Can you work these out from the model? Positions are in its coordinate system, mm. A direction names the side the tool comes from. Give positions to 0.01 mm unless a question says otherwise; leave off trailing zeros. Write each loop counter-clockwise with the first axis right and the second up, starting at its lowest first coordinate (ties: lowest second). Pieces come first, ordered by that corner, then holes. Notation, with made-up numbers: (70, 0.25) -> (92, 0.25) arc R29 cw to (92, 22.25) -> close; hole circle Ø4 at (-5, -26). An arc over 180 degrees is marked (long way). Answer as CSV lines item,"result". Start each with the question number.
1. I'm going to push flat-ended pins straight in: P1, Ø12, axis at x = 3.5, y = -3, coming from the -Z side; P2, Ø12, axis at x = -11.5, z = -21.5, coming from the -Y side; P3, Ø2.5, axis at x = 5.5, z = 1, coming from the +Y side. Where does each tip first touch, or does it pass through?
2. If we section it at D-D on y = -17.5: Write out the boundary of the cut face in (x, z) (3 decimals), plus the area to 3 significant figures.
3. If we mould it in two halves opening along Z, with no side actions, what happens to faces 6 (the face through (-1.032, 16.25, -11.226)), 7 (the face through (21.31, 0.73, -4.7)), 8 (the face through (18.573, -5.104, 1.565))? For each: pulls with the +Z half, pulls with the -Z half, needs draft (parallel to the pull), parting line crosses it, or undercut.
4. I need wall thicknesses on line 1 (Z direction, x = 0, y = 7.35) (3 decimals); line 2 (Z direction, x = 0, y = 18) (1 decimal); line 3 (Z direction, x = -15, y = -16) (3 decimals). Which ranges of each line are inside material? Lowest first, please. Write a range as [from, to].
5. On a 3-axis mill with a long thin cutter (end or side, diameter ignored), from which of +Z, -Z, +X, -X, +Y, -Y can I reach the whole of each face in a straight line? I mean faces 1 (the face through (0, -14, 0)), 2 (the face through (1, 8.458, -18.1)), 3 (the face through (0.49, 6.99, -13.68)), 4 (the face through (-19.05, 1, -1)), 5 (the face through (-0.33, 17.78, -31.44)). Say none if no direction works.
6. If we section it at A-A on x = 0: Count the separate pieces of the cut face and the enclosed holes in it, plus the area to 3 significant figures.
7. If we section it at B-B on y = 1: Write out the boundary of the cut face in (x, z) (3 decimals).
```python
from build123d import *
from build123d.topology import SkipClean

# Parameters (mm, degrees)
SKETCH1_R                                           = 23.8252
BOSS_EXTRUDE1_DEPTH                                 = 3.175
SKETCH8_W                                           = 38.1
SKETCH8_H                                           = 11.1125
CUT_EXTRUDE1_DEPTH                                  = 34.843181515
FILLET1_R                                           = 1.5875
BOSS_EXTRUDE2_START                                 = 31.75
BOSS_EXTRUDE2_DEPTH                                 = 31.75
CHAMFER1_START                                      = -23.8252001
CHAMFER1_DEPTH                                      = 6.3627001
CHAMFER1_START_2                                    = 17.4625
CHAMFER1_2_DEPTH                                    = 6.3627
CHAMFER1_START_3                                    = -31.7500001
CHAMFER1_3_DEPTH                                    = 31.7500001
CBORE_FOR_8_BINDING_HEAD_MACHINE_SCREW1_D           = 4.4958
CBORE_FOR_8_BINDING_HEAD_MACHINE_SCREW1_CBORE_D     = 9.525
CBORE_FOR_8_BINDING_HEAD_MACHINE_SCREW1_CBORE_DEPTH = 15.367
CHAMFER3_SIZE                                       = 6.35


with BuildPart() as part:
    # Sketch1 → Boss-Extrude1 (new body)
    with BuildSketch(Plane.XY):
        Circle(SKETCH1_R)
    extrude(amount=BOSS_EXTRUDE1_DEPTH)

    # Sketch8 → Cut-Extrude1 (cut, through all)
    with BuildSketch(Plane.XY.offset(3.175)):
        Rectangle(SKETCH8_W, SKETCH8_H)
    extrude(amount=-CUT_EXTRUDE1_DEPTH, mode=Mode.SUBTRACT)

    # Fillet1
    fillet1_edges = [part.edges().sort_by_distance(p)[0] for p in [
        (19.05, -5.55625, 1.5875),
        (-19.05, -5.55625, 1.5875),
        (-19.05, 5.55625, 1.5875),
        (19.05, 5.55625, 1.5875),
    ]]
    fillet(fillet1_edges, radius=FILLET1_R)

    # Sketch9 → Boss-Extrude2 (add)
    with SkipClean():  # the faces are left unmerged after this step: merging them gives an invalid solid
        with BuildSketch(Plane(origin=(0, 0, 0), x_dir=(-1, 0, 0), z_dir=(0, 0, -1)).offset(BOSS_EXTRUDE2_START)):
            with BuildLine():
                Line((-23.168259343, 5.55625), (23.168259343, 5.55625))
                ThreePointArc((23.168259343, 5.55625), (0, 23.8252), (-23.168259343, 5.55625))
            make_face()
        extrude(amount=-BOSS_EXTRUDE2_DEPTH)

    # Chamfer1: read off the stored shape, not the designer's step
    # Chamfer1 outline → Chamfer1 (add)
    with SkipClean():  # the faces are left unmerged after this step: merging them gives an invalid solid
        with BuildSketch(Plane.YZ.offset(CHAMFER1_START)):
            Polygon((5.55625, 0), (-3.96875, 0), (5.55625, -9.525), align=None)
        extrude(amount=CHAMFER1_DEPTH)

    # Chamfer1 2 outline → Chamfer1 2 (add)
    with SkipClean():  # the faces are left unmerged after this step: merging them gives an invalid solid
        with BuildSketch(Plane.YZ.offset(CHAMFER1_START_2)):
            Polygon((5.55625, 0), (-3.96875, 0), (5.55625, -9.525), align=None)
        extrude(amount=CHAMFER1_2_DEPTH)

    # Chamfer1 3 outline → Chamfer1 3 (cut)
    with BuildSketch(Plane.XY.offset(CHAMFER1_START_3)):
        with BuildLine():
            Line((23.8252, -5), (23.8252, 0))
            ThreePointArc((23.8252, 0), (23.692188185, -2.514035408), (23.294637903, -5))
            Line((23.294637903, -5), (23.8252, -5))
        make_face()
        with BuildLine():
            ThreePointArc((23.168259343, 5.55625), (23.660394835, 2.797475875), (23.8252, 0))
            Line((23.8252, 0), (23.8252, 5.55625))
            Line((23.8252, 5.55625), (23.168259343, 5.55625))
        make_face()
        with BuildLine():
            ThreePointArc((19.05, 3.96875), (18.585032015, 5.091282015), (17.4625, 5.55625))
            Line((17.4625, 5.55625), (17.4625, -5))
            Line((17.4625, -5), (19.05, -5))
            Line((19.05, -5), (19.05, 3.96875))
        make_face()
        with BuildLine():
            Line((-23.8252001, -5), (-23.294637903, -5))
            ThreePointArc((-23.294637903, -5), (-23.692188185, -2.514035408), (-23.8252, 0))
            Line((-23.8252, 0), (-23.8252001, -5))
        make_face()
        with BuildLine():
            Line((-17.4625, -5), (-17.4625, 5.55625))
            ThreePointArc((-17.4625, 5.55625), (-18.585032015, 5.091282015), (-19.05, 3.96875))
            Line((-19.05, 3.96875), (-19.05, -5))
            Line((-19.05, -5), (-17.4625, -5))
        make_face()
        with BuildLine():
            Line((-23.8252001, 5.55625), (-23.8252, 0))
            ThreePointArc((-23.8252, 0), (-23.660394835, 2.797475875), (-23.168259343, 5.55625))
            Line((-23.168259343, 5.55625), (-23.8252001, 5.55625))
        make_face()
    extrude(amount=CHAMFER1_3_DEPTH, mode=Mode.SUBTRACT)

    # CBORE for #8 Binding Head Machine Screw1 (through all)
    with Locations(Plane(origin=(0, 23.8252, 0), x_dir=(1, 0, 0), z_dir=(0, 1, 0))):
        with Locations((0, 15.875)):
            CounterBoreHole(CBORE_FOR_8_BINDING_HEAD_MACHINE_SCREW1_D / 2, CBORE_FOR_8_BINDING_HEAD_MACHINE_SCREW1_CBORE_D / 2, CBORE_FOR_8_BINDING_HEAD_MACHINE_SCREW1_CBORE_DEPTH)

    # Chamfer3
    chamfer3_edges = [part.edges().sort_by_distance(p)[0] for p in [
        (0, 23.8252, -31.75),
    ]]
    chamfer(chamfer3_edges, length=CHAMFER3_SIZE)


solid = part.part
```
Computed values:
1,P1,"stops at z = 0"
1,P2,"stops at y = 5.56"
1,P3,"stops at y = 23.44"
2,outline,"(-16.168, 0) -> (16.168, 0) -> (16.168, 3.175) -> (-16.168, 3.175) -> close"
2,area,"103 mm2"
3,face 6,"undercut"
3,face 7,"pulls with the -Z half"
3,face 8,"needs draft"
4,line 1,"z = [-31.75, -18.123], [-13.627, 3.175]"
4,line 2,"z = [-31.2, -20.6], [-11.1, 3.2]"
4,line 3,"z = [0, 3.175]"
5,face 1,"-Z, +X, -X, -Y"
5,face 2,"+Y"
5,face 3,"+Y, -Y"
5,face 4,"+Z, -Z"
5,face 5,"-Z, +Y"
6,separate pieces,"3"
6,enclosed holes,"0"
6,area,"516 mm2"
7,outline,"(-23.804, -4.969) -> (-19.05, -4.969) -> (-19.05, 3.175) -> (-23.804, 3.175) -> close; (19.05, -4.969) -> (23.804, -4.969) -> (23.804, 3.175) -> (19.05, 3.175) -> close"
